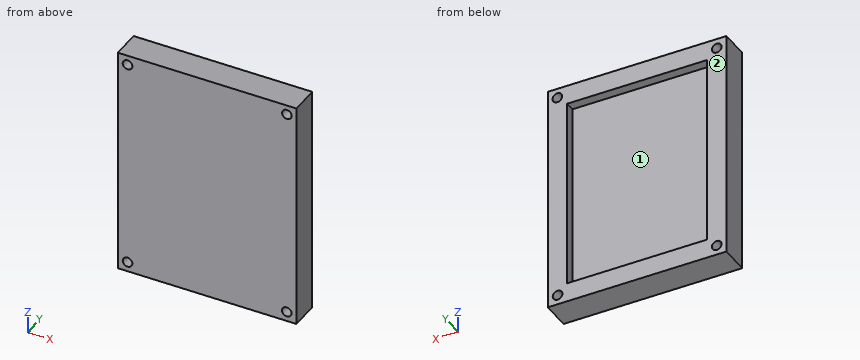
Autodesk Inventor part; units mm, degrees
ref_plane "YZ Plane" through (0, 0, 0) normal (1, 0, 0) x (0, 1, 0)
ref_plane "XZ Plane" through (0, 0, 0) normal (0, 1, 0) x (-1, 0, 0)
ref_plane "XY Plane" through (0, 0, 0) normal (0, 0, 1) x (1, 0, 0)
sketch "Sketch1" plane through (0, 0, 0) normal (0, 1, 0) x (-1, 0, 0)
  line L0 (0, 0) -> (92.5, 0)
  line L1 (92.5, 0) -> (92.5, -120)
  line L2 (92.5, -120) -> (0, -120)
  line L3 (0, -120) -> (0, 0)
  dimension "d0" = 120
  dimension "d1" = 92.5
extrude "Extrusion1" add sketch "Sketch1" along normal blind 15
shell "Shell1" thickness 10 removed faces 1 at (-30.8333, 15, -80)
sketch "Sketch3" plane through (0, 15, 0) normal (0, 1, 0) x (1, 0, 0)
  line L0 (-92.5, 0) -> (0, 0)
  line L1 (0, 0) -> (0, 4.953)
  line L2 (0, 0) -> (0, 120)
  line L3 (-4.953, 4.953) -> (0, 4.953)
  line L4 (-4.953, 4.953) -> (-4.953, 0)
  dimension "d5" = 4.953
  dimension "d6" = 4.953
hole "Hole1" at (-4.953, 15, -4.953) direction (0, -1, 0) diameter 5 end through all
sketch "Sketch5" plane through (0, 15, 0) normal (0, 1, 0) x (1, 0, 0)
  line L0 (-82.5, 10) -> (-82.5, 110)
  line L1 (-82.5, 10) -> (-87.453, 10)
  line L2 (-87.453, 10) -> (-87.453, 5.047)
  point P0 (0, 0)
  dimension "d14" = 4.953
  dimension "d15" = 4.953
hole "Hole2" at (-87.453, 15, -5.047) direction (0, -1, 0) diameter 5 end through all
sketch "Sketch6" plane through (0, 15, 0) normal (0, 1, 0) x (1, 0, 0)
  line L0 (-82.5, 110) -> (-10, 110)
  line L1 (-82.5, 110) -> (-82.5, 114.953)
  line L2 (-82.5, 114.953) -> (-87.453, 114.953)
  point P0 (0, 0)
  dimension "d23" = 4.953
  dimension "d24" = 4.953
hole "Hole3" at (-87.453, 15, -114.953) direction (0, -1, 0) diameter 5 end through all
sketch "Sketch7" plane through (0, 15, 0) normal (0, 1, 0) x (1, 0, 0)
  line L0 (-82.5, 110) -> (-10, 110)
  line L1 (-10, 110) -> (-10, 114.953)
  line L2 (-10, 114.953) -> (-5.047, 114.953)
  point P0 (0, 0)
  dimension "d32" = 4.953
  dimension "d33" = 4.953
hole "Hole4" at (-5.047, 15, -114.953) direction (0, -1, 0) diameter 5 end through all
properties part number "Water_Proof_Box_Top"
Verification items for the finished model (mm, model axes). Face numbers are marked on the shaded views. Coordinates: 2 decimals unless noted, no trailing zeros. Order: outer loops, then holes, each group sorted by start corner. A loop starts at its lowest first (then second) coordinate and runs counter-clockwise, first axis right, second up.
1. Sectioned sample at A-A, the plane z = -60.5. Record the cut outline in (x, y), and give its area (4 significant figures).
Results found:
outline: (-92.5, 0) - (0, 0) - (0, 15) - (-10, 15) - (-10, 10) - (-82.5, 10) - (-82.5, 15) - (-92.5, 15) - close
area: 1,025 mm2
2. Go/stop test with a flat-tipped pin: pin 1 Ø22 at (x, z) = (-30, -45) entering from +Y. Record where the tip stops, or that it passes through.
Results found:
pin 1: stops at y = 10
3. Scan lines: line 1 (Z direction, x = -31, y = 11.5); line 2 (X direction, y = 11.5, z = -18); line 3 (X direction, y = 3.25, z = -6). Record each from-to range of solid material in increasing order.
Results found:
line 1: z = -120 to -110, -10 to 0
line 2: x = -92.5 to -82.5, -10 to 0
line 3: x = -92.5 to -89.76, -85.14 to -7.22, -2.68 to 0
4. Sectioned sample at C-C, the plane x = -60. Record the cut outline in (y, z).
Results found:
outline: (0, -120) - (15, -120) - (15, -110) - (10, -110) - (10, -10) - (15, -10) - (15, 0) - (0, 0) - close
5. Release check for a two-part mould opening along X. For the marked faces 1 and 2 record: +X half, -X half, draft (parallel to the pull), parting line (faces both ways), or undercut.
Results found:
face 1: undercut
face 2: draft
6. Sectioned sample at B-B, the plane y = 12.5. Record the cut outline in (x, z).
Results found:
outline: (-92.5, -120) - (0, -120) - (0, 0) - (-92.5, 0) - close; hole circle Ø5 at (-87.45, -114.95); hole circle Ø5 at (-87.45, -5.05); hole (-82.5, -110) - (-10, -110) - (-10, -10) - (-82.5, -10) - close; hole circle Ø5 at (-5.05, -114.95); hole circle Ø5 at (-4.95, -4.95)
